The model under review builds one solid part; all positions refer to its coordinate system, in mm. Face numbers are marked on the shaded views. A direction names the side the tool comes from. Give positions to 0.01 mm unless a question says otherwise; leave off trailing zeros. Loops run counter-clockwise (first coordinate to the right, second up) from the corner with the lowest first, then second, coordinate; pieces in that order, holes last. Notation, with made-up numbers: M 30,-29.75 L 50,-29.75 A15 ccw 50,-23.75 Z; hole C 65,10.5 d4. An arc over 180 degrees is marked long. One line per item, written item: value. Start each with the question number.
Q1. We need section A-A on x = 40. Write out the cut boundary in (y, z), plus the area to 3 significant figures.
Q2. We need section B-B on y = 21.5. Write out the cut boundary in (x, z).
Q3. For the marked faces 1 and 2, list the 3-axis set-ups (+Z, -Z, +X, -X, +Y, -Y) from which the entire face can be reached by the end or side of a thin tool; tool diameter is ignored.
Q4. We need section C-C on x = -11.5. Write out the cut boundary in (y, z), plus the area to 3 significant figures.
Q5. To check wall thickness, follow line 1 along X through (y, z) = (12, 7); line 2 along X through (y, z) = (16, 7.25); line 3 along X through (y, z) = (5, 4). State the ranges of each line that lie inside material, in increasing order. Write a range as from..to.
Q6. For pin 1 (1 mm diameter, centred on y = 42.5, z = 5, fed in from -X); pin 2 (1.5 mm diameter, centred on y = -36, z = 4, fed in from -X); pin 3 (3 mm diameter, centred on x = -35.5, z = 6.5, fed in from -Y), all flat-tipped, find the tip position at first contact; note any pin that passes through.
Q7. We need section D-D on x = -43. Write out the cut boundary in (y, z), plus the area to 3 significant figures.
Q8. Mouldability with a two-part tool opening along Y and no side actions: class the marked faces 3, 4 and 5 as released by +Y, released by -Y, zero draft, split by the parting line, or undercut.
```python
from build123d import *
from OCP.BRepAlgoAPI import BRepAlgoAPI_Cut
from OCP.TopTools import TopTools_ListOfShape
from build123d.topology import SkipClean

# Parameters (mm, degrees)
BOSS_EXTRUDE1_DEPTH = 7.5
CUT_EXTRUDE1_DEPTH  = 3.2
CUT_EXTRUDE4_REACH  = 70.655
SKETCH5_W           = 3
SKETCH5_H           = 17
CUT_EXTRUDE5_REACH  = 70.655
SKETCH8_W           = 12
SKETCH8_H           = 37
CUT_EXTRUDE6_DEPTH  = 3.2
SKETCH10_W          = 10
SKETCH10_H          = 7.5
BOSS_EXTRUDE2_DEPTH = 27.486353186
SKETCH11_W          = 3
SKETCH11_H          = 7.5
CUT_EXTRUDE7_DEPTH  = 3.5
SKETCH12_W          = 2
SKETCH12_H          = 7.5
CUT_EXTRUDE8_DEPTH  = 4
SKETCH13_W          = 2
SKETCH13_H          = 7.5
CUT_EXTRUDE9_DEPTH  = 4
SKETCH14_W          = 7.5
SKETCH14_H          = 9.5
CUT_EXTRUDE10_DEPTH = 6
SKETCH15_W          = 1.5
SKETCH15_H          = 21
SKETCH15_H_2        = 1
CUT_EXTRUDE11_DEPTH = 1.5
SKETCH16_W          = 1.5
SKETCH16_H          = 7.5
CUT_EXTRUDE12_DEPTH = 35.486360958
CUT_EXTRUDE13_DEPTH = 6


with BuildPart() as part:
    # Sketch1 → Boss-Extrude1 (new body)
    with BuildSketch(Plane.XY):
        with BuildLine():
            Line((-33, -47.5), (49, -47.5))
            Line((49, -47.5), (49, -29.5))
            Line((49, -29.5), (31.5, -29.5))
            Line((31.5, -29.5), (31.5, 2.5))
            Line((31.5, 2.5), (49, 2.5))
            Line((49, 2.5), (49, 47.5))
            Line((49, 47.5), (30, 47.5))
            Line((30, 47.5), (30, 30.5))
            Line((30, 30.5), (27, 30.5))
            Line((27, 30.5), (27, 47.5))
            Line((27, 47.5), (-49, 47.5))
            Line((-49, 47.5), (-49, -31.5))
            ThreePointArc((-49, -31.5), (-44.313708499, -42.813708499), (-33, -47.5))
        make_face()
    extrude(amount=BOSS_EXTRUDE1_DEPTH)

    # Sketch2 → Cut-Extrude1 (cut)
    with BuildSketch(Plane.XY.offset(7.5)):
        Polygon((30, 40), (31, 40), (31, 32.5), (36, 32.5), (36, 28.5), (38, 28.5), (38, 32.5), (48, 32.5), (48, 46.5), (38, 46.5), (38, 47.5), (36, 47.5), (36, 46.5), (31, 46.5), (31, 45), (30, 45), align=None)
        Polygon((-16, 40), (-15, 40), (-15, 32.5), (-10, 32.5), (-10, 28.5), (-8, 28.5), (-8, 32.5), (2, 32.5), (2, 46.5), (-8, 46.5), (-8, 47.5), (-10, 47.5), (-10, 46.5), (-15, 46.5), (-15, 45), (-16, 45), align=None)
        Polygon((7, 40), (8, 40), (8, 32.5), (13, 32.5), (13, 28.5), (15, 28.5), (15, 32.5), (25, 32.5), (25, 46.5), (15, 46.5), (15, 47.5), (13, 47.5), (13, 46.5), (8, 46.5), (8, 45), (7, 45), align=None)
    extrude(amount=-CUT_EXTRUDE1_DEPTH, mode=Mode.SUBTRACT)

    # Sketch5 → Cut-Extrude4 (cut, up to next)
    with BuildSketch(Plane.XY.offset(7.5), mode=Mode.PRIVATE) as cut_extrude4_sk1:
        with Locations((5.5, 39)):
            Rectangle(SKETCH5_W, SKETCH5_H)
    cut_extrude4_tool1 = extrude(cut_extrude4_sk1.sketch, amount=-CUT_EXTRUDE4_REACH, mode=Mode.PRIVATE) & part.part
    # Sketch5 → Cut-Extrude4 (cut, up to next)
    with BuildSketch(Plane.XY.offset(7.5), mode=Mode.PRIVATE) as cut_extrude4_sk2:
        with Locations((-17.5, 39)):
            Rectangle(SKETCH5_W, SKETCH5_H)
    cut_extrude4_tool2 = extrude(cut_extrude4_sk2.sketch, amount=-CUT_EXTRUDE4_REACH, mode=Mode.PRIVATE) & part.part
    add(cut_extrude4_tool1.solids().sort_by_distance((5.5, 39, 7.5))[0], mode=Mode.SUBTRACT)
    add(cut_extrude4_tool2.solids().sort_by_distance((-17.5, 39, 7.5))[0], mode=Mode.SUBTRACT)

    # Sketch8 → Cut-Extrude5 (cut, up to next)
    with BuildSketch(Plane.XY.offset(7.5), mode=Mode.PRIVATE) as cut_extrude5_sk1:
        with Locations((-43, 29)):
            Rectangle(SKETCH8_W, SKETCH8_H)
    cut_extrude5_tool1 = extrude(cut_extrude5_sk1.sketch, amount=-CUT_EXTRUDE5_REACH, mode=Mode.PRIVATE) & part.part
    add(cut_extrude5_tool1.solids().sort_by_distance((-43, 29, 7.5))[0], mode=Mode.SUBTRACT)

    # Sketch9 → Cut-Extrude6 (cut)
    with BuildSketch(Plane.XY.offset(7.5)):
        Polygon((-37, 20), (-36, 20), (-36, 12.5), (-31, 12.5), (-31, 8.5), (-29, 8.5), (-29, 12.5), (-19, 12.5), (-19, 26.5), (-29, 26.5), (-29, 30.5), (-31, 30.5), (-31, 26.5), (-36, 26.5), (-36, 25), (-37, 25), align=None)
    extrude(amount=-CUT_EXTRUDE6_DEPTH, mode=Mode.SUBTRACT)

    # Sketch10 → Boss-Extrude2 (add)
    with BuildSketch(Plane(origin=(0, 10.5, 0), x_dir=(1, 0, 0), z_dir=(0, 1, 0))):
        with Locations((-44, -3.75)):
            Rectangle(SKETCH10_W, SKETCH10_H)
    extrude(amount=BOSS_EXTRUDE2_DEPTH)

    # Sketch11 → Cut-Extrude7 (cut)
    with BuildSketch(Plane(origin=(0, 30.5, 0), x_dir=(1, 0, 0), z_dir=(0, 1, 0))):
        with Locations((-17.5, -3.75)):
            Rectangle(SKETCH11_W, SKETCH11_H)
        with Locations((5.5, -3.75)):
            Rectangle(SKETCH11_W, SKETCH11_H)
        with Locations((28.5, -3.75)):
            Rectangle(SKETCH11_W, SKETCH11_H)
    extrude(amount=-CUT_EXTRUDE7_DEPTH, mode=Mode.SUBTRACT)

    # Sketch12 → Cut-Extrude8 (cut)
    with BuildSketch(Plane(origin=(0, 10.5, 0), x_dir=(1, 0, 0), z_dir=(0, 1, 0))):
        with Locations((-38, -3.75)):
            Rectangle(SKETCH12_W, SKETCH12_H)
    extrude(amount=-CUT_EXTRUDE8_DEPTH, mode=Mode.SUBTRACT)

    # Sketch13 → Cut-Extrude9 (cut)
    with BuildSketch(Plane(origin=(0, 6.5, 0), x_dir=(1, 0, 0), z_dir=(0, 1, 0))):
        with Locations((-38, -3.75)):
            Rectangle(SKETCH13_W, SKETCH13_H)
    extrude(amount=-CUT_EXTRUDE9_DEPTH, mode=Mode.SUBTRACT)

    # Sketch14 → Cut-Extrude10 (cut)
    with BuildSketch(Plane.ZY.offset(37)):
        with Locations((3.75, 42.75)):
            Rectangle(SKETCH14_W, SKETCH14_H)
    extrude(amount=-CUT_EXTRUDE10_DEPTH, mode=Mode.SUBTRACT)

    # Sketch15 → Cut-Extrude11 (cut)
    with BuildSketch(Plane.XY.offset(7.5)):
        with Locations((-19.75, 37)):
            Rectangle(SKETCH15_W, SKETCH15_H)
        with Locations((1.25, 47)):
            Rectangle(SKETCH15_W, SKETCH15_H_2)
        with Locations((24.25, 47)):
            Rectangle(SKETCH15_W, SKETCH15_H_2)
        with Locations((47.25, 47)):
            Rectangle(SKETCH15_W, SKETCH15_H_2)
    extrude(amount=-CUT_EXTRUDE11_DEPTH, mode=Mode.SUBTRACT)


with BuildPart() as cut_extrude12_tool:
    # Sketch16 → Cut-Extrude12 (new body)
    with BuildSketch(Plane(origin=(0, 37.986353186, 0), x_dir=(1, 0, 0), z_dir=(0, 1, 0))):
        with Locations((-39.75, -3.75)):
            Rectangle(SKETCH16_W, SKETCH16_H)
    extrude(amount=-CUT_EXTRUDE12_DEPTH)


with BuildPart() as part_1:
    add(part.part)

    # Cut-Extrude12: cut by cut_extrude12_tool, with a tolerance
    cut_extrude12_stock = TopTools_ListOfShape()
    cut_extrude12_stock.Append(part_1.part.wrapped)
    cut_extrude12_tools = TopTools_ListOfShape()
    cut_extrude12_tools.Append(cut_extrude12_tool.part.wrapped)
    cut_extrude12_cut = BRepAlgoAPI_Cut()
    cut_extrude12_cut.SetArguments(cut_extrude12_stock)
    cut_extrude12_cut.SetTools(cut_extrude12_tools)
    cut_extrude12_cut.SetFuzzyValue(0.00001)
    cut_extrude12_cut.Build()
    add(Compound.cast(cut_extrude12_cut.Shape()).solids(), mode=Mode.REPLACE)

    # Sketch18 → Cut-Extrude13 (cut)
    with SkipClean():  # the faces are left unmerged after this step: merging them gives an invalid solid
        with BuildSketch(Plane.XY.offset(7.5)):
            Polygon((23.5, 6.5), (23.5, 2.5), (46, 2.5), (46, 24), (49, 24), (49, 26), (46, 26), (23.5, 26), (23.5, 8.8), (18.5, 8.8), (18.5, 6.5), align=None)
        extrude(amount=-CUT_EXTRUDE13_DEPTH, mode=Mode.SUBTRACT)


solid = part_1.part
```
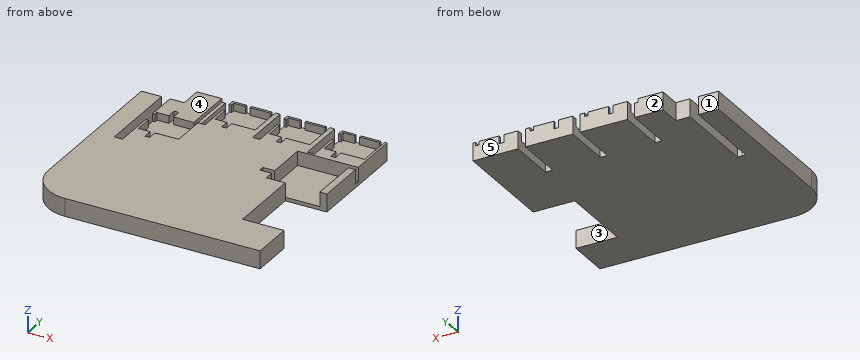
Solved:
1. outline: M -47.5,0 L -29.5,0 L -29.5,7.5 L -47.5,7.5 Z; M 2.5,0 L 47.5,0 L 47.5,7.5 L 46.5,7.5 L 46.5,4.3 L 32.5,4.3 L 32.5,7.5 L 26,7.5 L 26,1.5 L 2.5,1.5 Z
1. area: 287 mm2
2. outline: M -49,0 L -40.5,0 L -40.5,7.5 L -49,7.5 Z; M -37,0 L 49,0 L 49,7.5 L 46,7.5 L 46,1.5 L 23.5,1.5 L 23.5,7.5 L -19,7.5 L -19,4.3 L -37,4.3 Z
3. face 1: +Z, -Z, -X, +Y
3. face 2: +Z, -Z, +X, -X, +Y
4. outline: M -47.5,0 L 47.5,0 L 47.5,7.5 L 46.5,7.5 L 46.5,4.3 L 32.5,4.3 L 32.5,7.5 L -47.5,7.5 Z
4. area: 668 mm2
5. line 1: -49..-40.5, -37..-31, -29..23.5, 46..49
5. line 2: -49..-40.5, -37..-36, -19..23.5, 46..49
5. line 3: -49..-40.5, -37..23.5, 46..49
6. pin 1: x = -31
6. pin 2: x = -48.55
6. pin 3: y = -47.47
7. outline: M -43.99,0 L 37.99,0 L 37.99,7.5 L -43.99,7.5 Z
7. area: 615 mm2
8. face 3: undercut
8. face 4: zero draft
8. face 5: released by +Y
